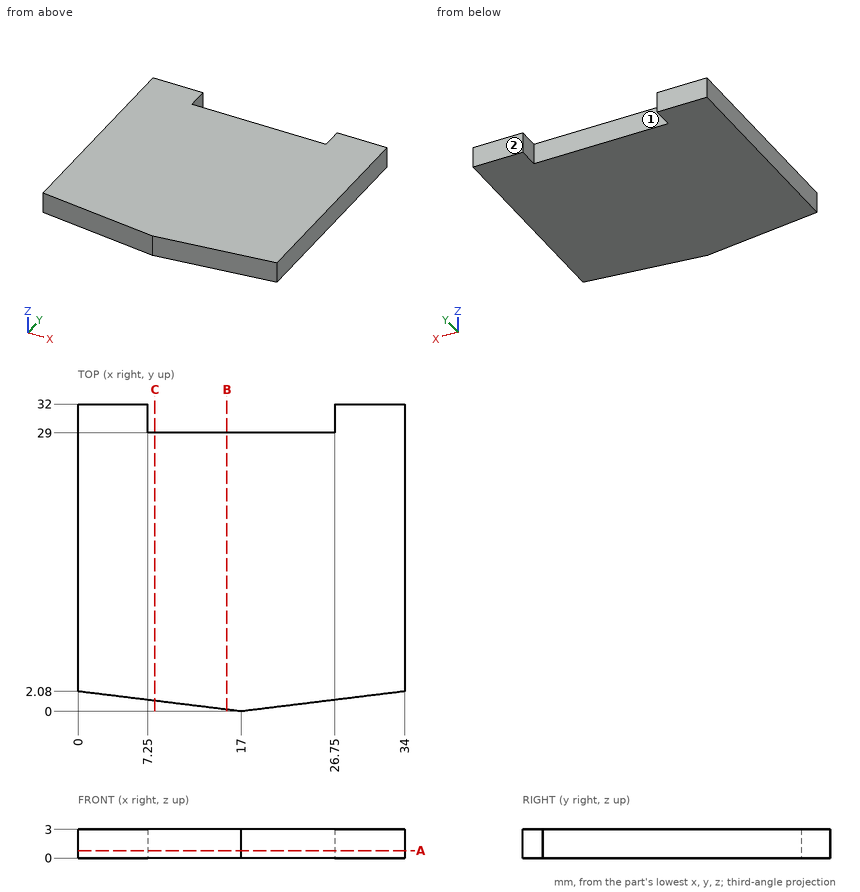
Answer from the drawing. Dimensions are ordinates in mm from the lowest x, y and z of the part. A direction names the side the tool comes from. Round coordinates to 2 decimals unless told otherwise and drop trailing zeros. Order: outer loops, then holes, each group sorted by start corner. A loop starts at its lowest first (then second) coordinate and runs counter-clockwise, first axis right, second up. Notation, with made-up numbers: (-7.75, -24) - (41.25, -24) arc R32 cw to (41.25, 12) - close; hole circle Ø2 at (47.5, 1). An arc over 180 degrees is marked (long way). Put each result on its own line as item: value. Start each with the question number.
(1) Straight lines are drawn through the part: probe 1 along Y at (x, z) = (18.5, 0.3); probe 2 along Y at (x, z) = (12, 2.1). For each, find the intervals that lie inside material, in ascending order. Write a range as from..to.
(2) Find section C-C (x = 8). Give the vertices of the cut face in (y, z).
(3) Find section A-A (z = 0.8). Give the vertices of the cut face in (x, y), plus the area to 3 significant figures.
(4) For the marked faces 1 and 2, determine the directions among +Z, -Z, +X, -X, +Y, -Y from which every point of the face is accessible in a straight line to the end or side of a thin tool.
(5) Find section B-B (x = 15.5). Give the vertices of the cut face in (y, z).
(6) Given P1, Ø1.5, axis at x = 14, z = 0.5, coming from the +Y side, flat-ended and moving along its own axis, determine where the tip first touches the part or whether it passes through.
Reply:
1. probe 1: 0.18..29
1. probe 2: 0.61..29
2. outline: (1.1, 0) - (29, 0) - (29, 3) - (1.1, 3) - close
3. outline: (0, 2.08) - (17, 0) - (34, 2.08) - (34, 32) - (26.75, 32) - (26.75, 29) - (7.25, 29) - (7.25, 32) - (0, 32) - close
3. area: 994 mm^2
4. face 1: +Z, -Z, +Y
4. face 2: +Z, -Z, +X, -X, +Y
5. outline: (0.18, 0) - (29, 0) - (29, 3) - (0.18, 3) - close
6. P1: y = 29
